from build123d import *

# Parameters (mm, degrees)
F0_R           = 17.5
F1_DEPTH       = 5
F2_R           = 5.75
F3_DEPTH       = 0.5
F5_D           = 5.5
F5_CSINK_D     = 11.5
F5_CSINK_ANGLE = 90
F6_R           = 0.5


with BuildPart() as f1:
    # F0 (on Top) → F1 (new body)
    with BuildSketch(Plane.XY):
        Circle(F0_R)
    extrude(amount=F1_DEPTH)

    # F2 (on face) → F3 (cut)
    with BuildSketch(Plane.XY.offset(5)):
        Circle(F2_R)
    extrude(amount=-F3_DEPTH, mode=Mode.SUBTRACT)

    # F5 (through all)
    with Locations(Plane.XY.offset(4.5)):
        with Locations((0, 0)):
            CounterSinkHole(F5_D / 2, F5_CSINK_D / 2, counter_sink_angle=F5_CSINK_ANGLE)

    # F6
    f6_edges = [f1.edges().sort_by_distance(p)[0] for p in [
        (-17.5, 0, 5),
        (-17.5, 0, 0),
    ]]
    fillet(f6_edges, radius=F6_R)


solid = f1.part
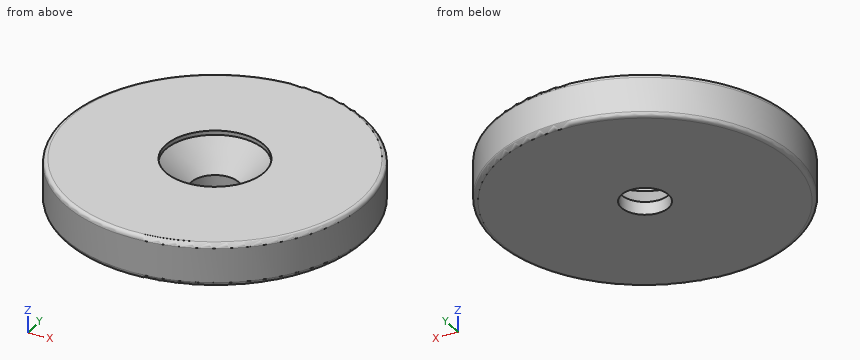
Verification items for the finished model (mm, model axes). Give positions to 0.01 mm unless a question says otherwise; leave off trailing zeros. Loops run counter-clockwise (first coordinate to the right, second up) from the corner with the lowest first, then second, coordinate; pieces in that order, holes last. Notation, with made-up numbers: (44, -26.5) - (96, -26.5) arc R16 ccw to (96, -14.5) - close; hole circle Ø2 at (38, -34.5). An arc over 180 degrees is marked (long way). Write each question's results on one line, items separated by ' | '.
1) Depth check by flat-ended pin: P1, Ø6.5, axis at x = 0, y = 0, coming from the +Z side; P2, Ø1.5, axis at x = 12.5, z = 1.5, coming from the +Y side. Enter the tip coordinate at first touch or a pass-through.
Solution:
P1: z = 2 | P2: y = 12.97
2) Material ranges on L1, parallel to Y at x = 0, z = 0.55; L2, parallel to Y at x = 0, z = 4.8; L3, parallel to X at y = -1, z = 3.3, recorded low to high. Write a range as from..to.
Solution:
L1: -17.5..-2.75, 2.75..17.5 | L2: -17.4..-5.75, 5.75..17.4 | L3: -17.47..-4.44, 4.44..17.47
3) Sectioned sample at A-A on x = 0. Record the boundary of the cut face in (y, z), plus the area to 3 significant figures.
Solution:
outline: (-17.5, 0.5) arc R0.5 ccw to (-17, 0) - (-2.75, 0) - (-2.75, 1.5) - (-5.75, 4.5) - (-5.75, 5) - (-17, 5) arc R0.5 ccw to (-17.5, 4.5) - close; (2.75, 0) - (17, 0) arc R0.5 ccw to (17.5, 0.5) - (17.5, 4.5) arc R0.5 ccw to (17, 5) - (5.75, 5) - (5.75, 4.5) - (2.75, 1.5) - close | area: 135 mm2
4) Sectioned sample at D-D on z = 2.95. Record the boundary of the cut face in (x, y).
Solution:
outline: circle Ø35 at (0, 0); hole circle Ø8.4 at (0, 0)
5) Sectioned sample at C-C on z = 1. Record the boundary of the cut face in (x, y), plus the area to 3 significant figures.
Solution:
outline: circle Ø35 at (0, 0); hole circle Ø5.5 at (0, 0) | area: 938 mm2
